Work out the finished part from the listing and answer in its coordinate system (mm). Give positions to 0.01 mm unless a question says otherwise; leave off trailing zeros. Loops run counter-clockwise (first coordinate to the right, second up) from the corner with the lowest first, then second, coordinate; pieces in that order, holes last. Notation, with made-up numbers: (-19, 79) - (-12, 79) arc R12 ccw to (-12, 89) - close; hole circle Ø5 at (71, -15). An arc over 180 degrees is marked (long way). Use CSV: the item, a comma, the result in double quotes.
from build123d import *

# Parameters (mm, degrees)
SKETCH1_W           = 35
SKETCH1_H           = 28
SKETCH1_R           = 2
BOSS_EXTRUDE1_DEPTH = 18
SKETCH2_R           = 4
CUT_EXTRUDE1_DEPTH  = 43.721340305


with BuildPart() as part:
    # Sketch1 → Boss-Extrude1 (new body)
    with BuildSketch(Plane.XY):
        with Locations((-13.540903953, 5.778964085)):
            Rectangle(SKETCH1_W, SKETCH1_H)
        with Locations((-25.540903953, 14.278964085)):
            Circle(SKETCH1_R, mode=Mode.SUBTRACT)
        with Locations((-1.540903953, 14.278964085)):
            Circle(SKETCH1_R, mode=Mode.SUBTRACT)
        with Locations((-25.540903953, -2.721035915)):
            Circle(SKETCH1_R, mode=Mode.SUBTRACT)
        with Locations((-1.540903953, -2.721035915)):
            Circle(SKETCH1_R, mode=Mode.SUBTRACT)
    extrude(amount=BOSS_EXTRUDE1_DEPTH)

    # Sketch2 → Cut-Extrude1 (cut, through all)
    with BuildSketch(Plane(origin=(-4.261939868, -8.221035915, 0), x_dir=(0, 0, -1), z_dir=(0, 1, 0))):
        with Locations(Location((-9, 9.278964085, 0), (0, 0, 180))):
            Circle(SKETCH2_R)
    extrude(amount=CUT_EXTRUDE1_DEPTH, mode=Mode.SUBTRACT)


solid = part.part
Item 1: The mould has two halves that part along X. Classify faces 1 (the flat face through (-31.041, 6, 9)), 2 (the flat face through (3.959, 6, 9)), 3 (the cylindrical face through (0.3, -3.5, 8.9)): pulls with the +X half, pulls with the -X half, needs draft (parallel to the pull), parting line crosses it, or undercut.
Determined:
face 1,"pulls with the -X half"
face 2,"pulls with the +X half"
face 3,"undercut"
Item 2: A cutting plane is placed at A-A on z = 9. Determine the outline of the cut face in (x, y).
Determined:
outline,"(-31.04, -8.22) - (-17.54, -8.22) - (-17.54, 19.78) - (-31.04, 19.78) - close; (-9.54, -8.22) - (3.96, -8.22) - (3.96, 19.78) - (-9.54, 19.78) - close; hole circle Ø4 at (-25.54, -2.72); hole circle Ø4 at (-25.54, 14.28); hole circle Ø4 at (-1.54, -2.72); hole circle Ø4 at (-1.54, 14.28)"
Item 3: A cutting plane is placed at D-D on y = 9. Determine the outline of the cut face in (x, z), and give its area (3 significant figures).
Determined:
outline,"(-31.04, 0) - (3.96, 0) - (3.96, 18) - (-31.04, 18) - close; hole circle Ø8 at (-13.54, 9)"
area,"580 mm²"
Item 4: A cutting plane is placed at B-B on x = -24.5. Determine the outline of the cut face in (y, z).
Determined:
outline,"(-8.22, 0) - (-4.43, 0) - (-4.43, 18) - (-8.22, 18) - close; (-1.01, 0) - (12.57, 0) - (12.57, 18) - (-1.01, 18) - close; (15.99, 0) - (19.78, 0) - (19.78, 18) - (15.99, 18) - close"
Item 5: Find the intervals of material crossed by line 1 (X direction, y = -4.25, z = 12.5); line 2 (X direction, y = -1.5, z = 8.75); line 3 (X direction, y = 18, z = 8.25), in increasing order.
Determined:
line 1,"x = -31.04 to -26.83, -24.25 to -15.48, -11.6 to -2.83, -0.25 to 3.96"
line 2,"x = -31.04 to -27.12, -23.96 to -17.53, -9.55 to -3.12, 0.04 to 3.96"
line 3,"x = -31.04 to -17.47, -9.61 to 3.96"
Item 6: A cutting plane is placed at C-C on z = 3. Determine the outline of the cut face in (x, y), and give its area (3 significant figures).
Determined:
outline,"(-31.04, -8.22) - (3.96, -8.22) - (3.96, 19.78) - (-31.04, 19.78) - close; hole circle Ø4 at (-25.54, -2.72); hole circle Ø4 at (-25.54, 14.28); hole circle Ø4 at (-1.54, -2.72); hole circle Ø4 at (-1.54, 14.28)"
area,"930 mm²"
